For this review, take the finished solid that the model builds, in its own axes (mm). A direction names the side the tool comes from. Coordinates: 2 decimals unless noted, no trailing zeros. Loops run counter-clockwise (first coordinate to the right, second up) from the corner with the lowest first, then second, coordinate; pieces in that order, holes last. Notation, with made-up numbers: (44.25, 8) -> (59.25, 8) arc R16 cw to (59.25, 14) -> close; hole circle Ø10 at (46, 28.25). An arc over 180 degrees is marked (long way). One line per item, written item: value.
from build123d import *

# Parameters (mm, degrees)
SKETCH1_W           = 180
SKETCH1_H           = 60
BOSS_EXTRUDE1_DEPTH = 1.2
SKETCH3_W           = 180
SKETCH3_H           = 60
SKETCH3_W_2         = 177.6
SKETCH3_H_2         = 57.6
BOSS_EXTRUDE2_DEPTH = 32
SKETCH4_W           = 40
SKETCH4_H           = 0.8
BOSS_EXTRUDE3_DEPTH = 10


with BuildPart() as part:
    # Sketch1 → Boss-Extrude1 (new body)
    with BuildSketch(Plane(origin=(0, 0, 0), x_dir=(1, 0, 0), z_dir=(0, 1, 0))):
        with Locations((90, 30)):
            Rectangle(SKETCH1_W, SKETCH1_H)
    extrude(amount=BOSS_EXTRUDE1_DEPTH)

    # Sketch3 → Boss-Extrude2 (add)
    with BuildSketch(Plane(origin=(0, 1.2, 0), x_dir=(1, 0, 0), z_dir=(0, 1, 0))):
        with Locations((90, 30)):
            Rectangle(SKETCH3_W, SKETCH3_H)
        with Locations((90, 30)):
            Rectangle(SKETCH3_W_2, SKETCH3_H_2, mode=Mode.SUBTRACT)
    extrude(amount=BOSS_EXTRUDE2_DEPTH)

    # Sketch4 → Boss-Extrude3 (add)
    with BuildSketch(Plane(origin=(0, 1.2, 0), x_dir=(1, 0, 0), z_dir=(0, 1, 0))):
        with Locations((36.2, 7.9)):
            Rectangle(SKETCH4_W, SKETCH4_H)
    extrude(amount=BOSS_EXTRUDE3_DEPTH)


solid = part.part
1. Take a section at A-A, the plane y = 9.5. Give the boundary of the cut face in (x, z), and give its area (3 significant figures).
Return value:
outline: (0, -60) -> (180, -60) -> (180, 0) -> (0, 0) -> close; (16.2, -8.3) -> (56.2, -8.3) -> (56.2, -7.5) -> (16.2, -7.5) -> close; hole (1.2, -58.8) -> (178.8, -58.8) -> (178.8, -1.2) -> (1.2, -1.2) -> close
area: 602 mm2
2. The part is to be moulded in two halves that separate along Z. For faces 3 (the flat face through (178.8, 17, -30)), 4 (the flat face through (90, 33.2, -59)), 5 (the flat face through (89, 16, 0)), 6 (the flat face through (36, 6, -7.5)), say which applies: pulls with the +Z half, pulls with the -Z half, needs draft (parallel to the pull), parting line crosses it, or undercut.
Return value:
face 3: undercut
face 4: needs draft
face 5: pulls with the +Z half
face 6: undercut
3. Insertion check: pin 1 Ø0.9 at (x, z) = (31, -8) entering from +Y. The pin has a flat end and moves straight along its axis. Give the tip position at first contact, or say it passes through.
Return value:
pin 1: stops at y = 11.2
4. To check wall thickness, follow probe 1 along Z at (x, y) = (108, 4.5); probe 2 along X at (y, z) = (30, -20.5); probe 3 along Y at (x, z) = (150, -53.5). State the ranges of each line that lie inside material, in increasing order. Write a range as from..to.
Return value:
probe 1: z = -60..-58.8, -1.2..0
probe 2: x = 0..1.2, 178.8..180
probe 3: y = 0..1.2
5. Take a section at C-C, the plane y = 23.5. Give the boundary of the cut face in (x, z), and give its area (3 significant figures).
Return value:
outline: (0, -60) -> (180, -60) -> (180, 0) -> (0, 0) -> close; hole (1.2, -58.8) -> (178.8, -58.8) -> (178.8, -1.2) -> (1.2, -1.2) -> close
area: 570 mm2
6. Take a section at B-B, the plane x = 20. Give the boundary of the cut face in (y, z).
Return value:
outline: (0, -60) -> (33.2, -60) -> (33.2, -58.8) -> (1.2, -58.8) -> (1.2, -8.3) -> (11.2, -8.3) -> (11.2, -7.5) -> (1.2, -7.5) -> (1.2, -1.2) -> (33.2, -1.2) -> (33.2, 0) -> (0, 0) -> close
7. Take a section at D-D, the plane z = -34. Give the boundary of the cut face in (x, y).
Return value:
outline: (0, 0) -> (180, 0) -> (180, 33.2) -> (178.8, 33.2) -> (178.8, 1.2) -> (1.2, 1.2) -> (1.2, 33.2) -> (0, 33.2) -> close
8. For faces 1 (the flat face through (180, 16, -30)), 2 (the flat face through (1.2, 17, -30)), list the 3-axis set-ups (+Z, -Z, +X, -X, +Y, -Y) from which the entire face can be reached by the end or side of a thin tool; tool diameter is ignored.
Return value:
face 1: +Z, -Z, +X, +Y, -Y
face 2: +Y
